Design review of the part built by this model. Coordinates are the model's own, in mm. A direction names the side the tool comes from. Coordinates: 2 decimals unless noted, no trailing zeros. Loops run counter-clockwise (first coordinate to the right, second up) from the corner with the lowest first, then second, coordinate; pieces in that order, holes last. Notation, with made-up numbers: (52.5, 58.5) -> (110.5, 58.5) arc R16 cw to (110.5, 68.5) -> close; hole circle Ø8 at (88.25, 36.5). An arc over 180 degrees is marked (long way). Use a Markdown table: item, result. Add a question column.
Q1. Take a section at B-B on y = 9.5. Write out the cut boundary in (x, z), plus the area to 3 significant figures.
Q2. For faces 4 (the face through (0, 54.5, 0)), 5 (the face through (15, 50.9, -4)), 6 (the face through (-1, 52.3, -1)), 7 (the face through (15, 6, 0)), list the 3-axis set-ups (+Z, -Z, +X, -X, +Y, -Y) from which the entire face can be reached by the end or side of a thin tool; tool diameter is ignored.
Q3. Draft analysis for pull direction X (two halves, no side actions). For faces 1 (the face through (-17, 3, 0)), 2 (the face through (-0.2, 54.5, 3.4)), 3 (the face through (-0.424, 0.588, -12.605)), state which applies: pulls with the +X half, pulls with the -X half, needs draft (parallel to the pull), parting line crosses it, or undercut.
Q4. Take a section at A-A on y = 1.5. Write out the cut boundary in (x, z), plus the area to 3 significant figures.
Q5. Clearance check with flat-ended pins moving along their axes: pin 1 Ø0.7 at (x, z) = (14.5, -6.5) entering from -Y; pin 2 Ø0.9 at (x, z) = (7.5, 14) entering from -Y; pin 3 Ø8 at (y, z) = (22.5, 12) entering from +X; pin 4 Ø4 at (x, y) = (-7, -8) entering from +Z. State where each tip first meets the part, or that it passes through.
Q6. For probe 1 along Y at (x, z) = (16, -4.5); probe 2 along X at (y, z) = (53, 0); probe 3 along Y at (x, z) = (-4.5, 13.5), list the stretches that pass through material, from the lowest coordinate up.
from build123d import *

# Parameters (mm, degrees)
SKETCH_1_R          = 18.4
EXTRUDE_1_DEPTH     = 21.5
SKETCH_2_R          = 6
EXTRUDE_2_DEPTH     = 6
SKETCH_3_R          = 3
EXTRUDE_3_DEPTH     = 13.8
SKETCH_4_W          = 8.972007795
SKETCH_4_H          = 2.543787651
CUT_EXTRUDE_1_DEPTH = 12
SKETCH_6_R          = 1.5
CUT_EXTRUDE_2_DEPTH = 6
CUT_EXTRUDE_3_DEPTH = 0.72
SKETCH_8_R          = 16.5
EXTRUDE_4_DEPTH     = 33
SKETCH_10_W         = 7.5
SKETCH_10_H         = 18
EXTRUDE_5_DEPTH     = 18
SKETCH_11_W         = 16.4
SKETCH_11_H         = 5.9
CUT_EXTRUDE_4_DEPTH = 5
SKETCH_12_W         = 0.64
SKETCH_12_H         = 0.64
EXTRUDE_6_DEPTH     = 4.5
SKETCH_13_W         = 16.4
SKETCH_13_H         = 1.5
EXTRUDE_7_DEPTH     = 5
SKETCH_14_R         = 3
CUT_EXTRUDE_5_DEPTH = 2.2
SKETCH_15_R         = 1
EXTRUDE_8_DEPTH     = 2.2
CHAMFER_1_SIZE      = 0.7
FILLET_1_R          = 0.3
FILLET_2_R          = 0.3


with BuildPart() as part:
    # 草图1 → 凸台-拉伸1 (new body)
    with BuildSketch(Plane(origin=(0, 0, 0), x_dir=(1, 0, 0), z_dir=(0, 1, 0))):
        Circle(SKETCH_1_R)
    extrude(amount=EXTRUDE_1_DEPTH)

    # 草图2 → 凸台-拉伸2 (add)
    with BuildSketch(Plane.XZ):
        with Locations((0, 7)):
            Circle(SKETCH_2_R)
    extrude(amount=EXTRUDE_2_DEPTH)

    # 草图3 → 凸台-拉伸3 (add)
    with BuildSketch(Plane.XZ.offset(6)):
        with Locations((0, 7)):
            Circle(SKETCH_3_R)
    extrude(amount=EXTRUDE_3_DEPTH)

    # 草图4 → 切除-拉伸1 (cut)
    with BuildSketch(Plane.XZ.offset(19.8)):
        with Locations((-0.051563263, 3.228106175)):
            Rectangle(SKETCH_4_W, SKETCH_4_H)
    extrude(amount=-CUT_EXTRUDE_1_DEPTH, mode=Mode.SUBTRACT)

    # 草图6 → 切除-拉伸2 (cut)
    with BuildSketch(Plane.XZ):
        with Locations((-15.5, 0)):
            Circle(SKETCH_6_R)
        with Locations((-7.75, 13.423393759)):
            Circle(SKETCH_6_R)
        with Locations((7.75, 13.423393759)):
            Circle(SKETCH_6_R)
        with Locations((15.5, 0)):
            Circle(SKETCH_6_R)
        with Locations((7.75, -13.423393759)):
            Circle(SKETCH_6_R)
        with Locations((-7.75, -13.423393759)):
            Circle(SKETCH_6_R)
    extrude(amount=-CUT_EXTRUDE_2_DEPTH, mode=Mode.SUBTRACT)

    # 草图7 → 切除-拉伸3 (cut)
    with BuildSketch(Plane.XZ):
        with BuildLine():
            ThreePointArc((-9.986582197, 7.517857143), (0, -12.5), (9.986582197, 7.517857143))
            ThreePointArc((9.986582197, 7.517857143), (0, -3), (-9.986582197, 7.517857143))
        make_face()
    extrude(amount=-CUT_EXTRUDE_3_DEPTH, mode=Mode.SUBTRACT)

    # 草图8 → 凸台-拉伸4 (add)
    with BuildSketch(Plane(origin=(0, 21.5, 0), x_dir=(1, 0, 0), z_dir=(0, 1, 0))):
        Circle(SKETCH_8_R)
    extrude(amount=EXTRUDE_4_DEPTH)

    # 草图10 → 凸台-拉伸5 (add)
    with BuildSketch(Plane(origin=(0, 0, 0), x_dir=(0, -1, 0), z_dir=(-0.984807753, 0, 0.173648178))):
        with Locations((-48.95, 0)):
            Rectangle(SKETCH_10_W, SKETCH_10_H)
    extrude(amount=-EXTRUDE_5_DEPTH)

    # 草图11 → 切除-拉伸4 (cut)
    with BuildSketch(Plane(origin=(17.726539554, 0, -3.125667198), x_dir=(-0.173648178, 0, -0.984807753), z_dir=(0.984807753, 0, -0.173648178))):
        with Locations((0, 48.95)):
            Rectangle(SKETCH_11_W, SKETCH_11_H)
    extrude(amount=-CUT_EXTRUDE_4_DEPTH, mode=Mode.SUBTRACT)

    # 草图12 → 凸台-拉伸6 (add)
    with BuildSketch(Plane(origin=(12.802500789, 0, -2.25742631), x_dir=(-0.173648178, 0, -0.984807753), z_dir=(0.984807753, 0, -0.173648178))):
        with Locations((-1.27, 50.58)):
            Rectangle(SKETCH_12_W, SKETCH_12_H)
        with Locations((1.27, 50.58)):
            Rectangle(SKETCH_12_W, SKETCH_12_H)
        with Locations((3.81, 50.58)):
            Rectangle(SKETCH_12_W, SKETCH_12_H)
        with Locations((6.35, 50.58)):
            Rectangle(SKETCH_12_W, SKETCH_12_H)
        with Locations((-6.35, 50.58)):
            Rectangle(SKETCH_12_W, SKETCH_12_H)
        with Locations((-3.81, 50.58)):
            Rectangle(SKETCH_12_W, SKETCH_12_H)
    extrude(amount=EXTRUDE_6_DEPTH)

    # 草图13 → 凸台-拉伸7 (add)
    with BuildSketch(Plane(origin=(12.802500789, 0, -2.25742631), x_dir=(-0.173648178, 0, -0.984807753), z_dir=(0.984807753, 0, -0.173648178))):
        with Locations((0, 46.75)):
            Rectangle(SKETCH_13_W, SKETCH_13_H)
    extrude(amount=EXTRUDE_7_DEPTH)

    # 草图14 → 切除-拉伸5 (cut)
    with BuildSketch(Plane(origin=(0, 54.5, 0), x_dir=(1, 0, 0), z_dir=(0, 1, 0))):
        Circle(SKETCH_14_R)
    extrude(amount=-CUT_EXTRUDE_5_DEPTH, mode=Mode.SUBTRACT)

    # 草图15 → 凸台-拉伸8 (add)
    with BuildSketch(Plane(origin=(0, 52.3, 0), x_dir=(1, 0, 0), z_dir=(0, 1, 0))):
        Circle(SKETCH_15_R)
    extrude(amount=EXTRUDE_8_DEPTH)

    # 倒角1
    chamfer_1_edges = [part.edges().sort_by_distance(p)[0] for p in [
        (0, 0, -12.5),
        (0, 0, -3),
    ]]
    chamfer(chamfer_1_edges, length=CHAMFER_1_SIZE)

    # 圆角1
    fillet_1_edges = [part.edges().sort_by_distance(p)[0] for p in [
        (-6, -6, 7),
    ]]
    fillet(fillet_1_edges, radius=FILLET_1_R)

    # 圆角2
    fillet_2_edges = [part.edges().sort_by_distance(p)[0] for p in [
        (-18.4, 0, 0),
        (-18.4, 21.5, 0),
    ]]
    fillet(fillet_2_edges, radius=FILLET_2_R)


solid = part.part
Answer list:
| question | item | result |
|---|---|---|
| 1 | outline | circle Ø36.8 at (0, 0) |
| 1 | area | 1,060 mm² |
| 2 | face 4 | +Z, -Z, +X, -X, +Y |
| 2 | face 5 | +X |
| 2 | face 6 | +Y |
| 2 | face 7 | -Y |
| 3 | face 1 | undercut |
| 3 | face 2 | needs draft |
| 3 | face 3 | undercut |
| 4 | outline | circle Ø36.8 at (0, 0); hole circle Ø3 at (-15.5, 0); hole circle Ø3 at (-7.75, -13.42); hole circle Ø3 at (-7.75, 13.42); hole circle Ø3 at (7.75, -13.42); hole circle Ø3 at (7.75, 13.42); hole circle Ø3 at (15.5, 0) |
| 4 | area | 1,020 mm² |
| 5 | pin 1 | y = 0 |
| 5 | pin 2 | y = 6 |
| 5 | pin 3 | x = 16.47 |
| 5 | pin 4 | through |
| 6 | probe 1 | 0 to 21.5, 45.2 to 47.5, 51.9 to 52.7 |
| 6 | probe 2 | -16.5 to -3, -1 to 1, 3 to 16.5 |
| 6 | probe 3 | 0 to 54.5 |
